Geometry: see drawing. Coordinates: mm, zero at the bounding-box minimum. Give positions to 0.01 mm unless a question says otherwise; leave off trailing zeros. Write each loop counter-clockwise with the first axis right and the second up, starting at its lowest first coordinate (ties: lowest second). Pieces come first, ordered by that corner, then holes. Notation, with made-up numbers: (-5.75, 29) -> (43.25, 29) arc R21 ccw to (43.25, 49) -> close; hole circle Ø6 at (49.5, -20.75). An arc over 180 degrees is marked (long way). Use one line per item in the form item = value. Start each with the question number.
(1) Cut plane A-A, the plane x = 3.25. Output: boundary loops of the cut face in (y, z), and give its area (3 significant figures).
(2) Cut plane B-B, the plane y = 3.5. Output: boundary loops of the cut face in (x, z) (3 decimals), and give its area (3 significant figures).
(3) Cut plane C-C, the plane x = 0.75. Output: boundary loops of the cut face in (y, z).
(4) First-contact query: P1, Ø2.5, axis at x = 3.175, z = 28.575, coming from the +Y side; P2, Ø3.5, axis at x = 3.175, z = 3.175, coming from the +Y side. Flat tips, straight axial feed; report the tip coordinate or a pass-through.
(5) Cut plane D-D, the plane x = 6. Output: boundary loops of the cut face in (y, z), and give its area (3 significant figures).
(6) Material intervals for line 1 along X through (y, z) = (2.7, 28); line 2 along Z through (x, y) = (4.5, 4.25); line 3 along Z through (x, y) = (2.5, 0.75), sorted ascending. Write a range as from..to.
(7) Draft query along X for the marked faces 1, 2 and 3. Return one class per face: pulls with the +X half, pulls with the -X half, needs draft (parallel to the pull), parting line crosses it, or undercut.
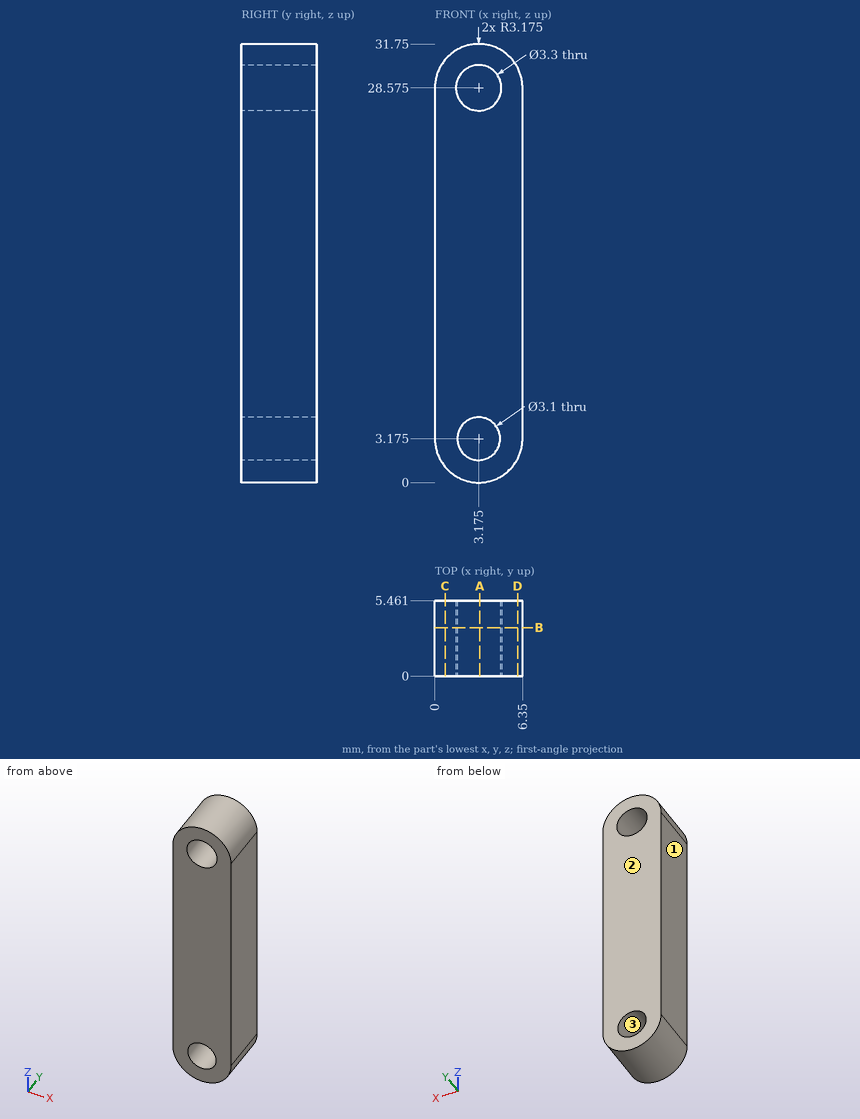
Geometry says:
q1.outline = (0, 0) -> (5.46, 0) -> (5.46, 1.63) -> (0, 1.63) -> close; (0, 4.72) -> (5.46, 4.72) -> (5.46, 26.93) -> (0, 26.93) -> close; (0, 30.22) -> (5.46, 30.22) -> (5.46, 31.75) -> (0, 31.75) -> close
q1.area = 138 mm^2
q2.outline = (0, 3.175) arc R3.175 ccw to (6.35, 3.175) -> (6.35, 28.575) arc R3.175 ccw to (0, 28.575) -> close; hole circle Ø3.3 at (3.175, 28.575); hole circle Ø3.1 at (3.175, 3.175)
q2.area = 177 mm^2
q3.outline = (0, 1.13) -> (5.46, 1.13) -> (5.46, 30.62) -> (0, 30.62) -> close
q4.P1 = through
q4.P2 = 5.46
q5.outline = (0, 1.73) -> (5.46, 1.73) -> (5.46, 30.02) -> (0, 30.02) -> close
q5.area = 155 mm^2
q6.line_1 = 0..1.63, 4.72..6.35
q6.line_2 = 0.29..2.37, 3.98..27.59, 29.56..31.46
q6.line_3 = 0.07..1.78, 4.57..27.07, 30.08..31.68
q7.face_1 = pulls with the -X half
q7.face_2 = needs draft
q7.face_3 = undercut
